Check sheet for the modelled part. Datum: model origin and axes. Units: mm. A direction names the side the tool comes from. Round coordinates to 2 decimals unless told otherwise and drop trailing zeros. Order: outer loops, then holes, each group sorted by start corner. A loop starts at its lowest first (then second) coordinate and runs counter-clockwise, first axis right, second up. Notation, with made-up numbers: (31, -1) -> (41, -1) arc R16 ccw to (41, 22) -> close; hole circle Ø11 at (4.25, 54). An arc over 180 degrees is marked (long way). Use CSV: the item, a comma, the result in double quotes.
```python
from build123d import *

# Parameters (mm, degrees)
SKETCH_1_W          = 157
SKETCH_1_H          = 47.4
EXTRUDE_1_DEPTH     = 36
FILLET_1_R          = 2
SKETCH_2_R          = 2
SKETCH_2_R_2        = 12
SKETCH_2_R_3        = 9
CUT_EXTRUDE_1_DEPTH = 20


with BuildPart() as part:
    # 草图1 → 凸台-拉伸1 (new body)
    with BuildSketch(Plane(origin=(0, 0, 0), x_dir=(1, 0, 0), z_dir=(0, 1, 0))):
        Rectangle(SKETCH_1_W, SKETCH_1_H)
    extrude(amount=EXTRUDE_1_DEPTH)

    # 圆角1
    fillet_1_edges = [part.edges().sort_by_distance(p)[0] for p in [
        (-78.5, 36, 0),
        (0, 36, 23.7),
        (78.5, 36, 0),
        (0, 0, 23.7),
        (-78.5, 0, 0),
        (0, 0, -23.7),
        (78.5, 0, 0),
        (78.5, 18, 23.7),
        (-78.5, 18, 23.7),
        (-78.5, 18, -23.7),
        (78.5, 18, -23.7),
        (0, 36, -23.7),
    ]]
    fillet(fillet_1_edges, radius=FILLET_1_R)

    # 草图2 → 切除-拉伸1 (cut)
    # profile 1 of 3: a face of its own
    with BuildSketch(Plane.XY.offset(23.7)):
        with Locations((0, 29)):
            Circle(SKETCH_2_R)
    # profile 2 of 3: a face of its own
    with BuildSketch(Plane.XY.offset(23.7)):
        with Locations((-58.5, 18)):
            Circle(SKETCH_2_R_2)
        with Locations((-58.5, 18)):
            Circle(SKETCH_2_R_3, mode=Mode.SUBTRACT)
    # profile 3 of 3: a face of its own
    with BuildSketch(Plane.XY.offset(23.7)):
        with Locations(Location((58.5, 18, 0), (0, 0, 180))):
            Circle(SKETCH_2_R_2)
        with Locations(Location((58.5, 18, 0), (0, 0, 180))):
            Circle(SKETCH_2_R_3, mode=Mode.SUBTRACT)
    extrude(amount=-CUT_EXTRUDE_1_DEPTH, mode=Mode.SUBTRACT)

    # 草图4 → 切除-旋转1 (revolve, cut)
    with BuildSketch(Plane(origin=(-58.5, 0, 0), x_dir=(0, -1, 0), z_dir=(-1, 0, 0)), mode=Mode.PRIVATE) as cut_revolve_1_sk:
        with BuildLine():
            Line((-18, 23.7), (-26, 23.7))
            Line((-26, 23.7), (-26, 22.302272637))
            ThreePointArc((-26, 22.302272637), (-22.037480816, 23.124288414), (-18, 23.4))
            Line((-18, 23.4), (-18, 23.7))
        make_face()
    cut_revolve_1 = revolve(cut_revolve_1_sk.sketch.rotate(Axis((-58.5, 18, 23.230858861), (0, 0, -1)), 180), axis=Axis((-58.5, 18, 23.230858861), (0, 0, -1)), mode=Mode.SUBTRACT)

    # 镜向1: 切除-旋转1 across plane
    add(cut_revolve_1.mirror(Plane(origin=(0, 0, 0), x_dir=(0, 0, 1), z_dir=(1, 0, 0))), mode=Mode.SUBTRACT)


solid = part.part
```
Q1. Go/stop test with a flat-tipped pin: pin 1 (9.5 mm diameter, centred on x = 58.5, y = 18, fed in from +Z). Record where the tip stops, or that it passes through.
Result sheet:
pin 1,"stops at z = 23.4"
Q2. Sectioned sample at B-B, the plane x = 0. Enter the section's corners in (y, z).
Result sheet:
outline,"(0, -21.7) arc R2 ccw to (2, -23.7) -> (34, -23.7) arc R2 ccw to (36, -21.7) -> (36, 21.7) arc R2 ccw to (34, 23.7) -> (31, 23.7) -> (31, 3.7) -> (27, 3.7) -> (27, 23.7) -> (2, 23.7) arc R2 ccw to (0, 21.7) -> close"
Q3. Sectioned sample at D-D, the plane x = 58.5. Enter the section's corners in (y, z).
Result sheet:
outline,"(0, -21.7) arc R2 ccw to (2, -23.7) -> (34, -23.7) arc R2 ccw to (36, -21.7) -> (36, 21.7) arc R2 ccw to (34, 23.7) -> (30, 23.7) -> (30, 3.7) -> (27, 3.7) -> (27, 23.7) -> (26, 23.7) -> (26, 22.3) arc R29.7 ccw to (10, 22.3) -> (10, 23.7) -> (9, 23.7) -> (9, 3.7) -> (6, 3.7) -> (6, 23.7) -> (2, 23.7) arc R2 ccw to (0, 21.7) -> close"
Q4. Access from +Z, -Z, +X, -X, +Y, -Y to the whole of each face (thin tool, end or side, straight path). Record for faces 1 (the face through (67.344, 9.89, 13.84)), 2 (the face through (-1, 18, 23.7)).
Result sheet:
face 1,"+Z"
face 2,"+Z, +X, -X, +Y, -Y"
Q5. Mould release check, pull along Y, two halves, no side actions. Record for faces 3 (the face through (54, 10, 3.7)), 4 (the face through (-1, 0, 0)), 5 (the face through (78.5, 18, 0)): pulls with the +Y half, pulls with the -Y half, needs draft (parallel to the pull), parting line crosses it, or undercut.
Result sheet:
face 3,"undercut"
face 4,"pulls with the -Y half"
face 5,"needs draft"
Q6. Sectioned sample at A-A, the plane z = 18. Enter the section's corners in (x, y), then the cut area to 3 significant figures.
Result sheet:
outline,"(-78.5, 2) arc R2 ccw to (-76.5, 0) -> (76.5, 0) arc R2 ccw to (78.5, 2) -> (78.5, 34) arc R2 ccw to (76.5, 36) -> (-76.5, 36) arc R2 ccw to (-78.5, 34) -> close; circle Ø18 at (-58.5, 18); circle Ø18 at (58.5, 18); hole circle Ø24 at (-58.5, 18); hole circle Ø4 at (0, 29); hole circle Ø24 at (58.5, 18)"
area,"5,240 mm^2"
Q7. Scan lines: L1, parallel to Y at x = 58, z = 13; L2, parallel to Y at x = 0, z = 11.25; L3, parallel to X at y = 23, z = 11. Record each from-to range of solid material in increasing order.
Result sheet:
L1,"y = 0 to 6.01, 9.01 to 26.99, 29.99 to 36"
L2,"y = 0 to 27, 31 to 36"
L3,"x = -78.5 to -69.41, -65.98 to -51.02, -47.59 to 47.59, 51.02 to 65.98, 69.41 to 78.5"
